Verification items for the finished model (mm, model axes). Face numbers are marked on the shaded views. A direction names the side the tool comes from. Coordinates: 2 decimals unless noted, no trailing zeros. Order: outer loops, then holes, each group sorted by start corner. A loop starts at its lowest first (then second) coordinate and runs counter-clockwise, first axis right, second up. Notation, with made-up numbers: (-28, -22) -> (26, -22) arc R16 cw to (26, -17) -> close; hole circle Ø8 at (-11.5, -40). An arc over 180 degrees is marked (long way). Write item = value, one per line. Start each with the question number.
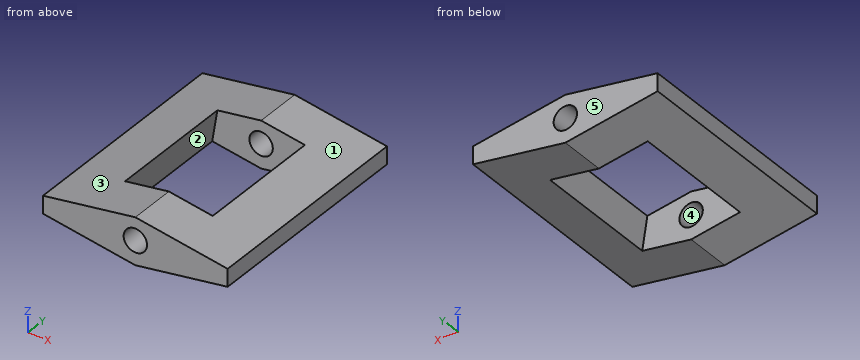
from build123d import *

# Parameters (mm, degrees)
F1_DEPTH = 120.65
F2_DEPTH = 120.65
F4_D     = 12.7
F6_W     = 26.88828125
F6_H     = 69.85
F7_DEPTH = 32.9290334674
F5_W     = 26.88828125
F5_H     = 69.85
F8_DEPTH = 32.9290334674


with BuildPart() as f1:
    # F0 (on Front) → F1 (new body)
    with BuildSketch(Plane.XZ):
        Polygon((-50.176050998, 0.6862330108), (-50.176050998, -8.8387669892), (0, -16.7762669892), (0, 8.6237330108), align=None)
    extrude(amount=F1_DEPTH)

    # F0 (on Front) → F2 (join)
    with BuildSketch(Plane.XZ):
        Polygon((0, 8.6237330108), (0, -16.7762669892), (50.176050998, -8.8387669892), (50.176050998, 0.6862330108), align=None)
    extrude(amount=F2_DEPTH)

    # F4 (through all)
    with Locations(Plane(origin=(0, 0, 0), x_dir=(1, 0, 0), z_dir=(0, 1, 0))):
        with Locations((0, 3.6785302916)):
            Hole(F4_D / 2)

    # F6 (on face) → F7 (cut, through all)
    with BuildSketch(Plane(origin=(-2.5890958046, 0, -16.3666901584), x_dir=(0.9877175393, 0, -0.15625), z_dir=(-0.15625, 0, -0.9877175393))):
        with Locations((-10.8228489079, 60.325)):
            Rectangle(F6_W, F6_H)
    extrude(amount=-F7_DEPTH, mode=Mode.SUBTRACT)

    # F5 (on face) → F8 (cut, through all)
    with BuildSketch(Plane(origin=(2.5890958046, 0, -16.3666901584), x_dir=(0.9877175393, 0, 0.15625), z_dir=(0.15625, 0, -0.9877175393))):
        with Locations((10.8228489079, 60.325)):
            Rectangle(F5_W, F5_H)
    extrude(amount=-F8_DEPTH, mode=Mode.SUBTRACT)


solid = f1.part
Item 1: Section check C-C (y = -20). Record the boundary of the cut face in (x, z).
Item 2: Mould release check, pull along X, two halves, no side actions. Record for the marked faces 3, 4 and 5: pulls with the +X half, pulls with the -X half, needs draft (parallel to the pull), parting line crosses it, or undercut.
Item 3: Section check B-B (z = -6.25). Record the boundary of the cut face in (x, y).
Item 4: Gauge pin test, flat ends, axial feed: P1, Ø1.5, axis at x = -7.5, y = -23, coming from the +Z side; P2, Ø5, axis at x = 35, y = -82.5, coming from the -Z side (3 decimals); P3, Ø6, axis at x = -12, y = -15.5, coming from the +Z side; P4, Ø2, axis at x = -39, z = -12.5, coming from the -Y side. Record the tip position at first contact, or that the pin passes through.
Item 5: Section check A-A (x = -9). Record the boundary of the cut face in (y, z), then the cut area to 3 significant figures.
Item 6: Section check D-D (x = 13.5). Record the boundary of the cut face in (y, z).
Item 7: Tool access check on the marked faces 1 and 2. Record the directions out of +Z, -Z, +X, -X, +Y, -Y that give a thin tool (end or side, any length) a straight path to the whole face; none if there is none.
Item 8: Thickness scan on line 1 (Z direction, x = 0, y = -11); line 2 (Y direction, x = 15, z = -6); line 3 (X direction, y = -19, z = -3.75). Record the ranges inside material, lowest first.
Filled sheet:
q1.outline = (-50.18, -8.84) -> (0, -16.78) -> (50.18, -8.84) -> (50.18, 0.69) -> (0, 8.62) -> (-50.18, 0.69) -> close; hole circle Ø12.7 at (0, -3.68)
q2.face_3 = pulls with the -X half
q2.face_4 = undercut
q2.face_5 = needs draft
q3.outline = (-50.18, -120.65) -> (-5.81, -120.65) -> (-5.81, -95.25) -> (-25.56, -95.25) -> (-25.56, -25.4) -> (-5.81, -25.4) -> (-5.81, 0) -> (-50.18, 0) -> close; (5.81, -120.65) -> (50.18, -120.65) -> (50.18, 0) -> (5.81, 0) -> (5.81, -25.4) -> (25.56, -25.4) -> (25.56, -95.25) -> (5.81, -95.25) -> close
q4.P1 = 7.56
q4.P2 = -11.635
q4.P3 = 7.2
q4.P4 = through
q5.outline = (-120.65, -15.35) -> (-95.25, -15.35) -> (-95.25, 7.2) -> (-120.65, 7.2) -> close; (-25.4, -15.35) -> (0, -15.35) -> (0, 7.2) -> (-25.4, 7.2) -> close
q5.area = 1,150 mm^2
q6.outline = (-120.65, -14.64) -> (-95.25, -14.64) -> (-95.25, 6.49) -> (-120.65, 6.49) -> close; (-25.4, -14.64) -> (0, -14.64) -> (0, 6.49) -> (-25.4, 6.49) -> close
q7.face_1 = +Z, +X, +Y, -Y
q7.face_2 = -Z
q8.line_1 = -16.78 to -10.03, 2.67 to 8.62
q8.line_2 = -120.65 to -95.25, -25.4 to 0
q8.line_3 = -50.18 to -6.35, 6.35 to 50.18
